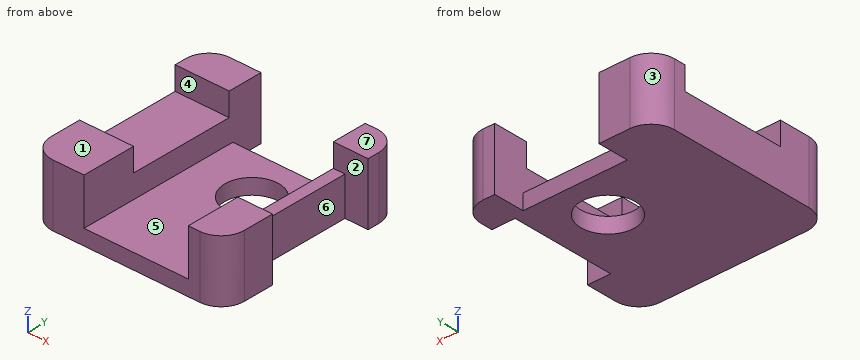
```python
from build123d import *

# Parameters (mm, degrees)
F0_W      = 25
F0_H      = 25
F1_DEPTH  = 8
F2_W      = 13.5
F2_H      = 25
F3_DEPTH  = 6
F4_R      = 3
F5_DEPTH  = 6
F6_W      = 7
F6_H      = 13.5
F7_DEPTH  = 3
F8_W      = 4.5
F8_H      = 13.5
F9_DEPTH  = 3
F10_W     = 3
F10_H     = 13.5
F11_DEPTH = 6
F12_W     = 13.5
F12_H     = 4
F13_DEPTH = 3
F15_D     = 7


with BuildPart() as f1:
    # F0 (on Top) → F1 (new body)
    with BuildSketch(Plane.XY):
        with Locations((-2.5, -2.5)):
            Rectangle(F0_W, F0_H)
    extrude(amount=F1_DEPTH)

    # F2 (on face) → F3 (cut)
    with BuildSketch(Plane.XY.offset(8)):
        with Locations((-1.25, -2.5)):
            Rectangle(F2_W, F2_H)
    extrude(amount=-F3_DEPTH, mode=Mode.SUBTRACT)

    # F4
    f4_edges = [f1.edges().sort_by_distance(p)[0] for p in [
        (10, -15, 4),
        (10, 10, 4),
        (-15, 10, 4),
        (-15, -15, 4),
    ]]
    fillet(f4_edges, radius=F4_R)

    # F2 (on face) → F5 (cut)
    with BuildSketch(Plane.XY.offset(8)):
        with Locations((-1.25, -2.5)):
            Rectangle(F2_W, F2_H)
    extrude(amount=-F5_DEPTH, mode=Mode.SUBTRACT)

    # F6 (on face) → F7 (cut)
    with BuildSketch(Plane.XY.offset(8)):
        with Locations((-11.5, -1.25)):
            Rectangle(F6_W, F6_H)
    extrude(amount=-F7_DEPTH, mode=Mode.SUBTRACT)

    # F8 (on face) → F9 (cut)
    with BuildSketch(Plane.XY.offset(8)):
        with Locations((7.75, -1.25)):
            Rectangle(F8_W, F8_H)
    extrude(amount=-F9_DEPTH, mode=Mode.SUBTRACT)

    # F10 (on face) → F11 (cut)
    with BuildSketch(Plane.XY.offset(5)):
        with Locations((8.5, -1.25)):
            Rectangle(F10_W, F10_H)
    extrude(amount=-F11_DEPTH, mode=Mode.SUBTRACT)

    # F12 (on face) → F13 (cut)
    with BuildSketch(Plane.XY.offset(2)):
        with Locations((-1.25, 8)):
            Rectangle(F12_W, F12_H)
    extrude(amount=-F13_DEPTH, mode=Mode.SUBTRACT)

    # F15 (through all)
    with Locations(Plane(origin=(0, 0, 0), x_dir=(1, 0, 0), z_dir=(0, 0, -1))):
        with Locations((0, 0)):
            Hole(F15_D / 2)


solid = f1.part
```
Work out the finished part from the listing and answer in its coordinate system (mm). Face numbers are marked on the shaded views. A direction names the side the tool comes from. Coordinates: 2 decimals unless noted, no trailing zeros. Loops run counter-clockwise (first coordinate to the right, second up) from the corner with the lowest first, then second, coordinate; pieces in that order, holes last. Notation, with made-up numbers: (78.5, 53.5) - (90.5, 53.5) arc R32 ccw to (90.5, 85.5) - close; hole circle Ø9 at (18, 7.5). An arc over 180 degrees is marked (long way). Use a Markdown table: item, result.
Item 1: Consider probe 1 along Y at (x, z) = (0, 1.5); probe 2 along X at (y, z) = (-10, 2.5). Determine where each line is inside the solid, lowest interval first. Write a range as from..to.
Evaluation:
| item | result |
|---|---|
| probe 1 | y = -15..-3.5, 3.5..6 |
| probe 2 | x = -15..-8, 5.5..10 |
Item 2: For the marked faces 4, 5, 6 and 7, determine the directions among +Z, -Z, +X, -X, +Y, -Y from which every point of the face is accessible in a straight line to the end or side of a thin tool.
Evaluation:
| item | result |
|---|---|
| face 4 | +Z, +X, -X |
| face 5 | +Z, +Y, -Y |
| face 6 | +Z, -Z, +X |
| face 7 | +Z, +X, -X, +Y, -Y |
Item 3: The mould has two halves that part along Y. Classify the marked faces 1, 2 and 3: +Y half, -Y half, draft (parallel to the pull), parting line (faces both ways), or undercut.
Evaluation:
| item | result |
|---|---|
| face 1 | draft |
| face 2 | undercut |
| face 3 | +Y half |
Item 4: Find section D-D, the plane z = 6. Determine the outline of the cut face in (x, y), and give its area (3 significant figures).
Evaluation:
| item | result |
|---|---|
| outline | (-15, -12) arc R3 ccw to (-12, -15) - (-8, -15) - (-8, -8) - (-15, -8) - close; (-15, 5.5) - (-8, 5.5) - (-8, 10) - (-12, 10) arc R3 ccw to (-15, 7) - close; (5.5, -15) - (7, -15) arc R3 ccw to (10, -12) - (10, -8) - (5.5, -8) - close; (5.5, 5.5) - (10, 5.5) - (10, 7) arc R3 ccw to (7, 10) - (5.5, 10) - close |
| area | 125 mm2 |
Item 5: Given pin 1 Ø5 at (x, y) = (-4.5, -1) entering from +Z; pin 2 Ø2 at (x, z) = (1.5, 1) entering from +Y; pin 3 Ø10 at (x, y) = (-7.5, -0.5) entering from -Z; pin 4 Ø5.5 at (x, y) = (-11, 0.5) entering from +Z, each flat-ended and moving along its own axis, determine where each tip first touches the part or whether it passes through.
Evaluation:
| item | result |
|---|---|
| pin 1 | stops at z = 2 |
| pin 2 | stops at y = 6 |
| pin 3 | stops at z = 0 |
| pin 4 | stops at z = 5 |
Item 6: Find section B-B, the plane z = 4.5. Determine the outline of the cut face in (x, y).
Evaluation:
| item | result |
|---|---|
| outline | (-15, -12) arc R3 ccw to (-12, -15) - (-8, -15) - (-8, 10) - (-12, 10) arc R3 ccw to (-15, 7) - close; (5.5, -15) - (7, -15) arc R3 ccw to (10, -12) - (10, -8) - (7, -8) - (7, 5.5) - (10, 5.5) - (10, 7) arc R3 ccw to (7, 10) - (5.5, 10) - close |
Item 7: Find section C-C, the plane x = 0. Determine the outline of the cut face in (y, z), and give its area (3 significant figures).
Evaluation:
| item | result |
|---|---|
| outline | (-15, 0) - (-3.5, 0) - (-3.5, 2) - (-15, 2) - close; (3.5, 0) - (6, 0) - (6, 2) - (3.5, 2) - close |
| area | 28.0 mm2 |
Item 8: Find section A-A, the plane y = 0. Determine the outline of the cut face in (x, z), and give its area (3 significant figures).
Evaluation:
| item | result |
|---|---|
| outline | (-15, 0) - (-3.5, 0) - (-3.5, 2) - (-8, 2) - (-8, 5) - (-15, 5) - close; (3.5, 0) - (7, 0) - (7, 5) - (5.5, 5) - (5.5, 2) - (3.5, 2) - close |
| area | 55.5 mm2 |
